Work out the finished part from the listing and answer in its coordinate system (mm). A direction names the side the tool comes from. Coordinates: 2 decimals unless noted, no trailing zeros. Loops run counter-clockwise (first coordinate to the right, second up) from the corner with the lowest first, then second, coordinate; pieces in that order, holes last. Notation, with made-up numbers: M 42.5,-32.5 L 78.5,-32.5 A32 ccw 78.5,0.5 Z; hole C 67.5,41 d4. An arc over 180 degrees is marked long. Write each question's results on one line, items separated by ' | '.
```python
from build123d import *

# Parameters (mm, degrees)
SKETCH_1_W          = 57
SKETCH_1_H          = 25
SKETCH_1_R          = 1.525
EXTRUDE_1_DEPTH     = 9
SKETCH_2_W          = 57
SKETCH_2_H          = 2
CUT_EXTRUDE_1_DEPTH = 3
SKETCH_3_W          = 40.5
SKETCH_3_H          = 20.3
CUT_EXTRUDE_2_DEPTH = 15
CUT_EXTRUDE_2_DRAFT = -2


with BuildPart() as part:
    # 草图1 → 凸台-拉伸1 (new body)
    with BuildSketch(Plane.XY):
        Rectangle(SKETCH_1_W, SKETCH_1_H)
        with Locations((24.3, 4.95)):
            Circle(SKETCH_1_R, mode=Mode.SUBTRACT)
        with Locations(Location((-24.3, 4.95, 0), (0, 0, 180))):
            Circle(SKETCH_1_R, mode=Mode.SUBTRACT)
        with Locations((-24.3, -4.95)):
            Circle(SKETCH_1_R, mode=Mode.SUBTRACT)
        with Locations(Location((24.3, -4.95, 0), (0, 0, 180))):
            Circle(SKETCH_1_R, mode=Mode.SUBTRACT)
    extrude(amount=EXTRUDE_1_DEPTH)

    # 草图2 → 切除-拉伸1 (cut)
    with BuildSketch(Plane.XY.offset(9)):
        Rectangle(SKETCH_2_W, SKETCH_2_H)
    extrude(amount=-CUT_EXTRUDE_1_DEPTH, mode=Mode.SUBTRACT)


with BuildPart() as cut_extrude_2_tool:
    # 草图3 → 切除-拉伸2 (with draft: the straight prism first)
    with BuildSketch(Plane.XY.offset(9)):
        Rectangle(SKETCH_3_W, SKETCH_3_H)
    extrude(amount=-CUT_EXTRUDE_2_DEPTH)
    # 切除-拉伸2: the draft: its side faces are tilted about the plane it starts from
    cut_extrude_2_sides = [cut_extrude_2_tool.faces().sort_by_distance(p)[0] for p in [
        (0, -10.15, 1.5),
        (20.25, 0, 1.5),
        (0, 10.15, 1.5),
        (-20.25, 0, 1.5),
    ]]
    draft(cut_extrude_2_sides, Plane.XY.offset(9), CUT_EXTRUDE_2_DRAFT)


with BuildPart() as part_1:
    add(part.part)

    # 切除-拉伸2: cut by cut_extrude_2_tool
    add(cut_extrude_2_tool.part, mode=Mode.SUBTRACT)


solid = part_1.part
```
1) Find section D-D, the plane z = 3. Give the vertices of the cut face in (x, y) (3 decimals), and give its area (3 significant figures).
Check result:
outline: M -28.5,-12.5 L 28.5,-12.5 L 28.5,12.5 L -28.5,12.5 Z; hole C -24.3,-4.95 d3.05; hole C -24.3,4.95 d3.05; hole M -20.04,-9.94 L 20.04,-9.94 L 20.04,9.94 L -20.04,9.94 Z; hole C 24.3,-4.95 d3.05; hole C 24.3,4.95 d3.05 | area: 599 mm^2
2) Find section C-C, the plane y = -7.5. Give the vertices of the cut face in (x, z), and give its area (3 significant figures).
Check result:
outline: M -28.5,0 L -19.94,0 L -20.25,9 L -28.5,9 Z; M 19.94,0 L 28.5,0 L 28.5,9 L 20.25,9 Z | area: 151 mm^2
3) Given pin 1 Ø1 at (x, y) = (23, 0) entering from +Z, flat-ended and moving along its own axis, determine where the tip first touches the part or whether it passes through.
Check result:
pin 1: z = 6
4) Find section A-A, the plane x = 24.3. Give the vertices of the cut face in (y, z) (3 decimals), and give its area (3 significant figures).
Check result:
outline: M -12.5,0 L -6.475,0 L -6.475,9 L -12.5,9 Z; M -3.425,0 L 3.425,0 L 3.425,9 L 1,9 L 1,6 L -1,6 L -1,9 L -3.425,9 Z; M 6.475,0 L 12.5,0 L 12.5,9 L 6.475,9 Z | area: 164 mm^2
5) For a pull along Y with two mould halves and no side action, classify faces 1 (the face through (24, 0, 6)), 2 (the face through (0, 12.5, 4)), 3 (the face through (-24, 1, 8)), 4 (the face through (0, -11, 9)) as released by +Y, released by -Y, zero draft, split by the parting line, or undercut.
Check result:
face 1: undercut | face 2: released by +Y | face 3: undercut | face 4: zero draft
6) Find section B-B, the plane y = -4.95. Give the vertices of the cut face in (x, z) (3 decimals), and give its area (3 significant figures).
Check result:
outline: M -28.5,0 L -25.825,0 L -25.825,9 L -28.5,9 Z; M -22.775,0 L -19.936,0 L -20.25,9 L -22.775,9 Z; M 19.936,0 L 22.775,0 L 22.775,9 L 20.25,9 Z; M 25.825,0 L 28.5,0 L 28.5,9 L 25.825,9 Z | area: 96.4 mm^2
7) Which of the six approach directions +Z, -Z, +X, -X, +Y, -Y give full straight-line access (tool end or side, diameter ignored) to faces 5 (the face through (28.5, 0, 4)), 6 (the face through (24, -1, 8))?
Check result:
face 5: +Z, -Z, +X, +Y, -Y | face 6: +Z, +X, -X
8) Straight lines are drawn through the part: probe 1 along Y at (x, z) = (-24.3, 5.25) (3 decimals); probe 2 along Y at (x, z) = (24.3, 6.25) (3 decimals); probe 3 along Y at (x, z) = (-25.5, 0.75). For each, find the intervals that lie inside material, in ascending order. Write a range as [from, to].
Check result:
probe 1: [-12.5, -6.475], [-3.425, 3.425], [6.475, 12.5] | probe 2: [-12.5, -6.475], [-3.425, -1], [1, 3.425], [6.475, 12.5] | probe 3: [-12.5, -5.89], [-4.01, 4.01], [5.89, 12.5]
